Read the model definition and answer for the solid it produces. Units are mm, in the model's axes. A direction names the side the tool comes from. Coordinates: 2 decimals unless noted, no trailing zeros. Loops run counter-clockwise (first coordinate to the right, second up) from the corner with the lowest first, then second, coordinate; pieces in that order, holes last. Notation, with made-up numbers: (-26, 33.5) -> (0, 33.5) arc R18 ccw to (0, 60.5) -> close; hole circle Ø2 at (32.25, -37.5). An arc over 180 degrees is marked (long way). Answer as CSV lines item,"result".
Autodesk Inventor part; units mm, degrees
ref_plane "YZ Plane" through (0, 0, 0) normal (1, 0, 0) x (0, 1, 0)
ref_plane "XZ Plane" through (0, 0, 0) normal (0, 1, 0) x (-1, 0, 0)
ref_plane "XY Plane" through (0, 0, 0) normal (0, 0, 1) x (1, 0, 0)
sketch "Sketch1" plane through (0, 0, 0) normal (0, 0, 1) x (1, 0, 0)
  circle A0 centre (0, 0) radius 5.1
  circle A1 centre (0, 0) radius 3.95
  circle A2 centre (0, 0) radius 3.15
  dimension "d0" = 10.2
  dimension "d1" = 7.9
  dimension "d4" = 6.3
extrude "Extrusion1" add sketch "Sketch1" along normal mid plane 10.3 contours A0 | A1
extrude "Extrusion2" add sketch "Sketch1" along normal mid plane 16.7 contours A1
properties part number "spacer" material "Stainless Steel"
Q1. For faces 4 (the face through (3, -3, -5.15)), 5 (the face through (-3, -2, -8.35)), determine the directions among +Z, -Z, +X, -X, +Y, -Y from which every point of the face is accessible in a straight line to the end or side of a thin tool.
Results:
face 4,"-Z"
face 5,"-Z, +X, -X, +Y, -Y"
Q2. Given pin 1 Ø5 at (x, y) = (0, 0.5) entering from +Z; pin 2 Ø1.5 at (x, y) = (4, 4) entering from -Z, each flat-ended and moving along its own axis, determine where each tip first touches the part or whether it passes through.
Results:
pin 1,"passes through"
pin 2,"stops at z = -5.15"
Q3. Find the intervals of material crossed by probe 1 along Y at (x, z) = (0, -3); probe 2 along Z at (x, y) = (-0.75, 4); probe 3 along X at (y, z) = (-0.25, -5.25), in increasing order. Write a range as [from, to].
Results:
probe 1,"y = [-5.1, -3.15], [3.15, 5.1]"
probe 2,"z = [-5.15, 5.15]"
probe 3,"x = [-3.94, -3.14], [3.14, 3.94]"
Q4. A cutting plane is placed at A-A, the plane x = 0. Write down the section's boundary in (y, z), and give its area (3 significant figures).
Results:
outline,"(-5.1, -5.15) -> (-3.95, -5.15) -> (-3.95, -8.35) -> (-3.15, -8.35) -> (-3.15, 8.35) -> (-3.95, 8.35) -> (-3.95, 5.15) -> (-5.1, 5.15) -> close; (3.15, -8.35) -> (3.95, -8.35) -> (3.95, -5.15) -> (5.1, -5.15) -> (5.1, 5.15) -> (3.95, 5.15) -> (3.95, 8.35) -> (3.15, 8.35) -> close"
area,"50.4 mm²"
Q5. For a pull along X with two mould halves and no side action, classify faces 1 (the face through (-2.5, -1.917, 0.117)), 2 (the face through (-3.135, 2.404, 6.728)), 3 (the face through (3, -3, 5.15)) as pulls with the +X half, pulls with the -X half, needs draft (parallel to the pull), parting line crosses it, or undercut.
Results:
face 1,"undercut"
face 2,"parting line crosses it"
face 3,"needs draft"
Q6. A cutting plane is placed at C-C, the plane z = -1. Write down the section's boundary in (x, y), and give its area (3 significant figures).
Results:
outline,"circle Ø10.2 at (0, 0); hole circle Ø6.3 at (0, 0)"
area,"50.5 mm²"
